```python
from build123d import *

# Parameters (mm, degrees)
ESQUISSE1_W             = 20
ESQUISSE1_H             = 8
BOSS_EXTRU_1_DEPTH      = 29
ESQUISSE2_R             = 7
ESQUISSE2_R_2           = 5
ENL_V_MAT_EXTRU_1_DEPTH = 70.728043139
ESQUISSE4_R             = 5
ENL_V_MAT_EXTRU_2_DEPTH = 62.002049146


with BuildPart() as part:
    # Esquisse1 → Boss.-Extru.1 (new body)
    with BuildSketch(Plane.XY):
        Polygon((0, 0), (30, 0), (30, 8), (30, 19.5), (0, 19.5), align=None)
        Polygon((30, -19.5), (30, -8), (30, 0), (0, 0), (0, -19.5), align=None)
        with Locations((40, -4)):
            Rectangle(ESQUISSE1_W, ESQUISSE1_H)
        with Locations((40, 4)):
            Rectangle(ESQUISSE1_W, ESQUISSE1_H)
    extrude(amount=BOSS_EXTRU_1_DEPTH)

    # Esquisse2 → Enlèv. mat.-Extru.1 (cut, through all)
    with BuildSketch(Plane(origin=(0, 19.5, 0), x_dir=(1, 0, 0), z_dir=(0, 1, 0))):
        with Locations(Location((15, -14.5, 0), (0, 0, 270))):
            Circle(ESQUISSE2_R)
        with Locations(Location((40, -14.5, 0), (0, 0, 270))):
            Circle(ESQUISSE2_R_2)
    extrude(amount=-ENL_V_MAT_EXTRU_1_DEPTH, mode=Mode.SUBTRACT)

    # Esquisse4 → Enlèv. mat.-Extru.2 (cut, through all)
    with BuildSketch(Plane.XY.offset(29)):
        with Locations((15, 0)):
            Circle(ESQUISSE4_R)
    extrude(amount=-ENL_V_MAT_EXTRU_2_DEPTH, mode=Mode.SUBTRACT)


solid = part.part
```
For this review, take the finished solid that the model builds, in its own axes (mm). A direction names the side the tool comes from. Give positions to 0.01 mm unless a question says otherwise; leave off trailing zeros. Write each loop counter-clockwise with the first axis right and the second up, starting at its lowest first coordinate (ties: lowest second). Pieces come first, ordered by that corner, then holes.
Item 1: The part is to be moulded in two halves that separate along Z. For faces 1 (the face through (44.216, 0.112, 17.188)), 2 (the face through (19, 5, 29)), 3 (the face through (19, 19.5, 8)), 4 (the face through (8.79, 0.27, 17.73)), say which applies: +Z half, -Z half, draft (parallel to the pull), parting line (faces both ways), or undercut.
Item 2: Take a section at B-B (x = 15). Give the boundary of the cut face in (y, z).
Item 3: Take a section at A-A (y = 0). Give the boundary of the cut face in (x, z), and give its area (3 significant figures).
Item 4: Take a section at C-C (x = 40). Give the boundary of the cut face in (y, z), and give its area (3 significant figures).
Item 5: Insertion check: P1, Ø9, axis at x = 15, y = 0, coming from the -Z side; P2, Ø6, axis at x = 38, z = 20, coming from the +Y side; P3, Ø6, axis at y = 12, z = 12.5, coming from the +X side; P4, Ø11.5, axis at x = 40, z = 14.5, coming from the -Y side. Each pin has a flat end and moves straight along its axis. Give the tip position at first contact, or say it passes through.
Item 6: Take a section at D-D (z = 23.25). Give the boundary of the cut face in (x, y), and give its area (3 significant figures).
Item 7: Machinability: for faces 5 (the face through (30, 14, 14)), 6 (the face through (19.77, 1.5, 3.8)), 7 (the face through (35, -8, 11)), which of the approach directions +Z, -Z, +X, -X, +Y, -Y give a long, thin tool a straight path to every point of the face, cutting with its end or side? Answer none if there is none.
Item 8: Wall thickness on probe 1 along X at (y, z) = (-2, 14.5); probe 2 along X at (y, z) = (0, 2.25); probe 3 along Z at (x, y) = (15, 9): over which ranges is each line inside the solid? List them lowest first.
Established:
1. face 1: undercut
1. face 2: +Z half
1. face 3: draft
1. face 4: undercut
2. outline: (-19.5, 0) - (-5, 0) - (-5, 7.5) - (-19.5, 7.5) - close; (-19.5, 21.5) - (-5, 21.5) - (-5, 29) - (-19.5, 29) - close; (5, 0) - (19.5, 0) - (19.5, 7.5) - (5, 7.5) - close; (5, 21.5) - (19.5, 21.5) - (19.5, 29) - (5, 29) - close
3. outline: (0, 0) - (10, 0) - (10, 9.6) arc R7 cw to (10, 19.4) - (10, 29) - (0, 29) - close; (20, 0) - (50, 0) - (50, 29) - (20, 29) - (20, 19.4) arc R7 cw to (20, 9.6) - close; hole circle Ø10 at (40, 14.5)
3. area: 1,050 mm2
4. outline: (-8, 0) - (8, 0) - (8, 9.5) - (-8, 9.5) - close; (-8, 19.5) - (8, 19.5) - (8, 29) - (-8, 29) - close
4. area: 304 mm2
5. P1: passes through
5. P2: stops at y = 8
5. P3: stops at x = 30
5. P4: stops at y = -8
6. outline: (0, -19.5) - (30, -19.5) - (30, -8) - (50, -8) - (50, 8) - (30, 8) - (30, 19.5) - (0, 19.5) - close; hole circle Ø10 at (15, 0)
6. area: 1,410 mm2
7. face 5: +Z, -Z, +X, +Y
7. face 6: +Z, -Z
7. face 7: +Z, -Z, +X, -Y
8. probe 1: x = 0 to 8, 22 to 35, 45 to 50
8. probe 2: x = 0 to 10, 20 to 50
8. probe 3: z = 0 to 7.5, 21.5 to 29
